from build123d import *

# Parameters (mm, degrees)
SKETCH_1_R      = 0.75
EXTRUDE_1_DEPTH = 3


with BuildPart() as part:
    # 草图1 → 凸台-拉伸1 (new body)
    with BuildSketch(Plane.XY):
        with BuildLine():
            Line((-10.5, 22.5), (-10.5, 13.638181697))
            ThreePointArc((-10.5, 13.638181697), (-7.5, 0), (-10.5, -13.638181697))
            Line((-10.5, -13.638181697), (-10.5, -22.5))
            ThreePointArc((-10.5, -22.5), (0, -33), (10.5, -22.5))
            Line((10.5, -22.5), (10.5, -13.638181697))
            ThreePointArc((10.5, -13.638181697), (7.5, 0), (10.5, 13.638181697))
            Line((10.5, 13.638181697), (10.5, 22.5))
            ThreePointArc((10.5, 22.5), (0, 33), (-10.5, 22.5))
        make_face()
        with Locations((6, 28.25)):
            Circle(SKETCH_1_R, mode=Mode.SUBTRACT)
        with Locations((-6, 28.25)):
            Circle(SKETCH_1_R, mode=Mode.SUBTRACT)
        with Locations((6, -28.25)):
            Circle(SKETCH_1_R, mode=Mode.SUBTRACT)
        with Locations((-6, -28.25)):
            Circle(SKETCH_1_R, mode=Mode.SUBTRACT)
        with BuildLine():
            ThreePointArc((4, 22.500000371), (-3.71e-07, 26.5), (-4, 22.499999629))
            Line((-4, 22.499999629), (-4, 8.5))
            Line((-4, 8.5), (4, 8.5))
            Line((4, 8.5), (4, 22.500000371))
        make_face(mode=Mode.SUBTRACT)
        with BuildLine():
            Line((4, -22.500000371), (4, -8.5))
            Line((4, -8.5), (-4, -8.5))
            Line((-4, -8.5), (-4, -22.499999629))
            ThreePointArc((-4, -22.499999629), (-3.71e-07, -26.5), (4, -22.500000371))
        make_face(mode=Mode.SUBTRACT)
    extrude(amount=EXTRUDE_1_DEPTH)


solid = part.part
Source: CAD feature listing. Evaluate the final solid. Frame: model axes, mm. A direction names the side the tool comes from. Round coordinates to 2 decimals unless told otherwise and drop trailing zeros. Write each loop counter-clockwise with the first axis right and the second up, starting at its lowest first coordinate (ties: lowest second). Pieces come first, ordered by that corner, then holes. Notation, with made-up numbers: (16.25, 36) - (52.25, 36) arc R34 cw to (52.25, 67) - close; hole circle Ø10 at (-19, -34). An arc over 180 degrees is marked (long way). Use CSV: the item, a comma, the result in double quotes. Start each with the question number.
(1) First-contact query: pin 1 Ø1 at (y, z) = (-3, 1) entering from +X; pin 2 Ø1.5 at (x, z) = (4.5, 1.5) entering from -Y; pin 3 Ø1 at (y, z) = (23.5, 1) entering from -X. Flat tips, straight axial feed; report the tip coordinate or a pass-through.
(2) Mould query, pull axis X, two halves, no side actions, for faces 3 (the face through (0, 33, 1)), 4 (the face through (10.5, -18, 1)), 5 (the face through (6, 29, 1)). Classes: pulls with the +X half, pulls with the -X half, needs draft (parallel to the pull), parting line crosses it, or undercut.
(3) Set-up query: faces 1 (the face through (-10.5, 18, 1)), 2 (the face through (-4, 16, 1)). Return all of +Z, -Z, +X, -X, +Y, -Y with unobstructed straight access to the full face (end or side cutting, diameter ignored); none if empty.
(4) Cut plane A-A, the plane z = 1.7. Return loops of the section in (x, y), and give its area (3 significant figures).
(5) Material intervals for probe 1 along X at (y, z) = (28, 0.4); probe 2 along Y at (x, z) = (-5.75, 2.55); probe 3 along Y at (x, z) = (-2, 0.8), sorted ascending. Write a range as [from, to].
(6) Cut plane B-B, the plane y = 28.25. Return loops of the section in (x, z).
(7) Cut plane C-C, the plane x = -6. Return loops of the section in (y, z), and give its area (3 significant figures).
(8) Cut plane D-D, the plane x = 9.25. Return loops of the section in (y, z).
Geometry says:
1,pin 1,"x = 7.69"
1,pin 2,"y = -32.31"
1,pin 3,"x = -10.49"
2,face 3,"parting line crosses it"
2,face 4,"pulls with the +X half"
2,face 5,"undercut"
3,face 1,"+Z, -Z, -X, +Y, -Y"
3,face 2,"+Z, -Z"
4,outline,"(-10.5, -22.5) arc R10.5 ccw to (10.5, -22.5) - (10.5, -13.64) arc R32.5 cw to (10.5, 13.64) - (10.5, 22.5) arc R10.5 ccw to (-10.5, 22.5) - (-10.5, 13.64) arc R32.5 cw to (-10.5, -13.64) - close; hole circle Ø1.5 at (-6, -28.25); hole circle Ø1.5 at (-6, 28.25); hole (-4, -22.5) arc R4 ccw to (4, -22.5) - (4, -8.5) - (-4, -8.5) - close; hole (-4, 8.5) - (4, 8.5) - (4, 22.5) arc R4 ccw to (-4, 22.5) - close; hole circle Ø1.5 at (6, -28.25); hole circle Ø1.5 at (6, 28.25)"
4,area,"900 mm²"
5,probe 1,"[-8.94, -6.71], [-5.29, 5.29], [6.71, 8.94]"
5,probe 2,"[-31.29, -28.96], [-27.54, 27.54], [28.96, 31.29]"
5,probe 3,"[-32.81, -25.96], [-8.5, 8.5], [25.96, 32.81]"
6,outline,"(-8.79, 0) - (-6.75, 0) - (-6.75, 3) - (-8.79, 3) - close; (-5.25, 0) - (5.25, 0) - (5.25, 3) - (-5.25, 3) - close; (6.75, 0) - (8.79, 0) - (8.79, 3) - (6.75, 3) - close"
7,outline,"(-31.12, 0) - (-29, 0) - (-29, 3) - (-31.12, 3) - close; (-27.5, 0) - (27.5, 0) - (27.5, 3) - (-27.5, 3) - close; (29, 0) - (31.12, 0) - (31.12, 3) - (29, 3) - close"
7,area,"178 mm²"
8,outline,"(-27.47, 0) - (-10.52, 0) - (-10.52, 3) - (-27.47, 3) - close; (10.52, 0) - (27.47, 0) - (27.47, 3) - (10.52, 3) - close"
